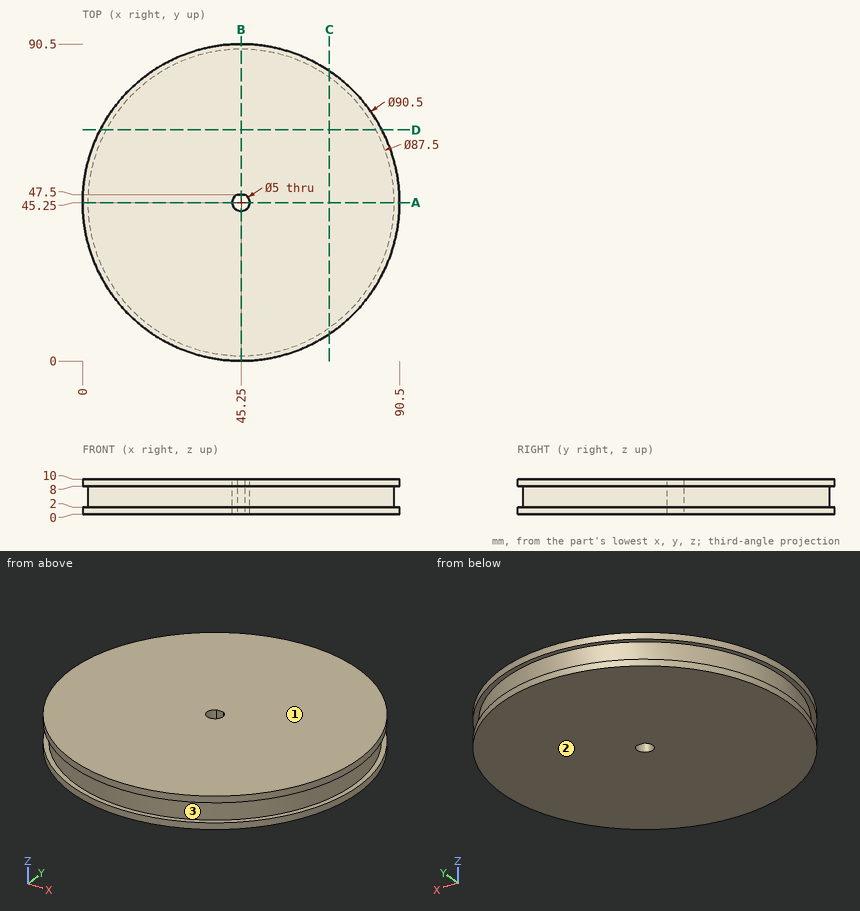
Geometry check sheet. Reference: drawing and pictorial views, mm from the part's lowest x, y, z. Coordinates: 2 decimals unless noted, no trailing zeros. Loops run counter-clockwise (first coordinate to the right, second up) from the corner with the lowest first, then second, coordinate; pieces in that order, holes last. Notation, with made-up numbers: M 77.25,-29.75 L 104.25,-29.75 A19 ccw 104.25,-20.75 Z; hole C 73.5,-12.75 d3. An arc over 180 degrees is marked long. One line per item, written item: value.
1. Section check A-A on y = 45.25. Record the cut outline in (x, z).
Answers follow:
outline: M 0,0 L 42.75,0 L 42.75,10 L 0,10 L 0,8 L 1.5,8 L 1.5,2 L 0,2 Z; M 47.75,0 L 90.5,0 L 90.5,2 L 89,2 L 89,8 L 90.5,8 L 90.5,10 L 47.75,10 Z
2. Section check C-C on x = 70.5. Record the cut outline in (y, z), plus the area to 3 significant figures.
Answers follow:
outline: M 7.7,0 L 82.8,0 L 82.8,2 L 80.98,2 L 80.98,8 L 82.8,8 L 82.8,10 L 7.7,10 L 7.7,8 L 9.52,8 L 9.52,2 L 7.7,2 Z
area: 729 mm^2
3. Material ranges on line 1 along Y through (x, z) = (45.25, 6); line 2 along Y through (x, z) = (45.5, 8.75); line 3 along X through (y, z) = (53.5, 0.75), recorded low to high. Write a range as from..to.
Answers follow:
line 1: 1.5..42.75, 47.5..89
line 2: 0..42.76, 47.5..90.5
line 3: 0.76..89.74
4. Section check B-B on x = 45.25. Record the cut outline in (y, z).
Answers follow:
outline: M 0,0 L 42.75,0 L 42.75,10 L 0,10 L 0,8 L 1.5,8 L 1.5,2 L 0,2 Z; M 47.5,0 L 90.5,0 L 90.5,2 L 89,2 L 89,8 L 90.5,8 L 90.5,10 L 47.5,10 Z
5. Mould release check, pull along Z, two halves, no side actions. Record for the marked faces 1, 2 and 3: pulls with the +Z half, pulls with the -Z half, needs draft (parallel to the pull), parting line crosses it, or undercut.
Answers follow:
face 1: pulls with the +Z half
face 2: pulls with the -Z half
face 3: undercut
6. Section check D-D on y = 66. Record the cut outline in (x, z).
Answers follow:
outline: M 5.04,0 L 85.46,0 L 85.46,2 L 83.77,2 L 83.77,8 L 85.46,8 L 85.46,10 L 5.04,10 L 5.04,8 L 6.73,8 L 6.73,2 L 5.04,2 Z
7. Gauge pin test, flat ends, axial feed: P1, Ø2, axis at x = 53.5, z = 4.5, coming from the -Y side; P2, Ø2, axis at y = 14.5, z = 5.5, coming from the -X side; P3, Ø4, axis at y = 53, z = 7, coming from the +X side. Record the tip position at first contact, or that the pin passes through.
Answers follow:
P1: y = 2.1
P2: x = 13.17
P3: x = 90.1
